```python
from build123d import *

# Parameters (mm, degrees)
F1_DEPTH = 101.6
F2_DEPTH = 67.564
F3_DEPTH = 33.782


with BuildPart() as f1:
    # F0 (on Front) → F1 (new body)
    with BuildSketch(Plane.XZ):
        Polygon((-24.286251, -20.083786), (77.313749, -20.083786), (77.313749, 0.464413), (39.213749, 0.464413), (13.813749, -8.153985), (-24.286251, -8.153985), align=None)
    extrude(amount=-F1_DEPTH)

    # F0 (on Front) → F2 (join)
    with BuildSketch(Plane.XZ):
        Polygon((39.213749, 0.464413), (77.313749, 0.464413), (77.313749, 8.618398), (39.213749, 8.618398), (13.813749, 0), (-24.286251, 0), (-24.286251, -8.153985), (13.813749, -8.153985), align=None)
    extrude(amount=-F2_DEPTH)

    # F0 (on Front) → F3 (join)
    with BuildSketch(Plane.XZ):
        Polygon((39.213749, 8.618398), (77.313749, 8.618398), (77.313749, 16.772382), (39.213749, 16.772382), (13.813749, 8.153985), (-24.286251, 8.153985), (-24.286251, 0), (13.813749, 0), align=None)
    extrude(amount=-F3_DEPTH)


solid = f1.part
```
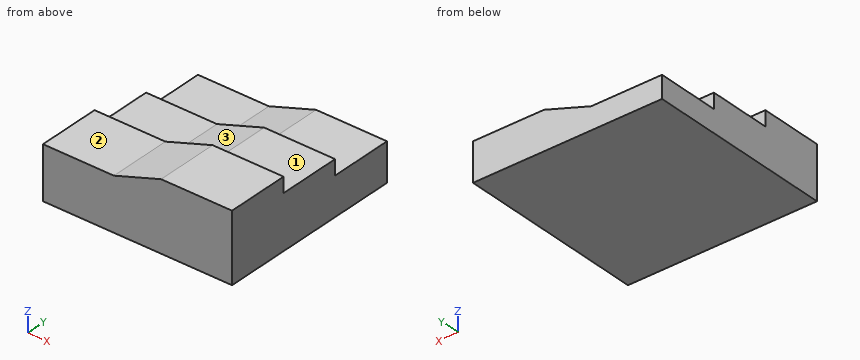
Geometry: final body of the model. Coordinates: model frame, mm. Face numbers are marked on the shaded views. A direction names the side the tool comes from. Give positions to 0.01 mm unless a question says otherwise; leave off trailing zeros. Loops run counter-clockwise (first coordinate to the right, second up) from the corner with the lowest first, then second, coordinate; pieces in that order, holes last. Notation, with made-up numbers: (73.5, 40) -> (127.5, 40) arc R14 cw to (127.5, 58) -> close; hole circle Ø4 at (39.25, 74). An arc over 180 degrees is marked (long way). Use one line per item in the form item = value.
Item 1: Section query A-A on x = 50.5. Output: boundary loops of the cut face in (y, z), and give its area (3 significant figures).
A:
outline = (0, -20.08) -> (101.6, -20.08) -> (101.6, 0.46) -> (67.56, 0.46) -> (67.56, 8.62) -> (33.78, 8.62) -> (33.78, 16.77) -> (0, 16.77) -> close
area = 2,910 mm^2
Item 2: Pin query (flat end, axial travel): P1, Ø8.5, axis at x = 52, z = 10, coming from the +Y side; P2, Ø10, axis at x = 67, y = 79, coming from the +Z side; P3, Ø10, axis at x = 2, z = 10.5, coming from the +Y side. Return the tip coordinate at first contact, or that it passes through.
A:
P1 = 67.56
P2 = 0.46
P3 = 33.78
Item 3: Section query B-B on y = 16. Output: boundary loops of the cut face in (x, z).
A:
outline = (-24.29, -20.08) -> (77.31, -20.08) -> (77.31, 16.77) -> (39.21, 16.77) -> (13.81, 8.15) -> (-24.29, 8.15) -> close
Item 4: Section query C-C on z = 6.5. Output: boundary loops of the cut face in (x, y), and give its area (3 significant figures).
A:
outline = (-24.29, 0) -> (77.31, 0) -> (77.31, 67.56) -> (32.97, 67.56) -> (32.97, 33.78) -> (-24.29, 33.78) -> close
area = 4,930 mm^2
Item 5: Access query for the marked faces 1, 2 and 3. Directions: +Z, -Z, +X, -X, +Y, -Y. A direction counts if a zero-diameter tool reaches every point of the face in a straight line with its end or side. Return the directions, or none.
A:
face_1 = +Z, +X, -X, +Y
face_2 = +Z, -X, +Y, -Y
face_3 = +Z, -X, +Y
Item 6: Section query D-D on x = -9.5. Output: boundary loops of the cut face in (y, z).
A:
outline = (0, -20.08) -> (101.6, -20.08) -> (101.6, -8.15) -> (67.56, -8.15) -> (67.56, 0) -> (33.78, 0) -> (33.78, 8.15) -> (0, 8.15) -> close
Item 7: Line query: probe 1 along Y at (x, z) = (69, 8); probe 2 along Z at (x, y) = (52.5, 71.5); probe 3 along Y at (x, z) = (3, 3). Output: solid intervals per line, ascending.
A:
probe_1 = 0 to 67.56
probe_2 = -20.08 to 0.46
probe_3 = 0 to 33.78
